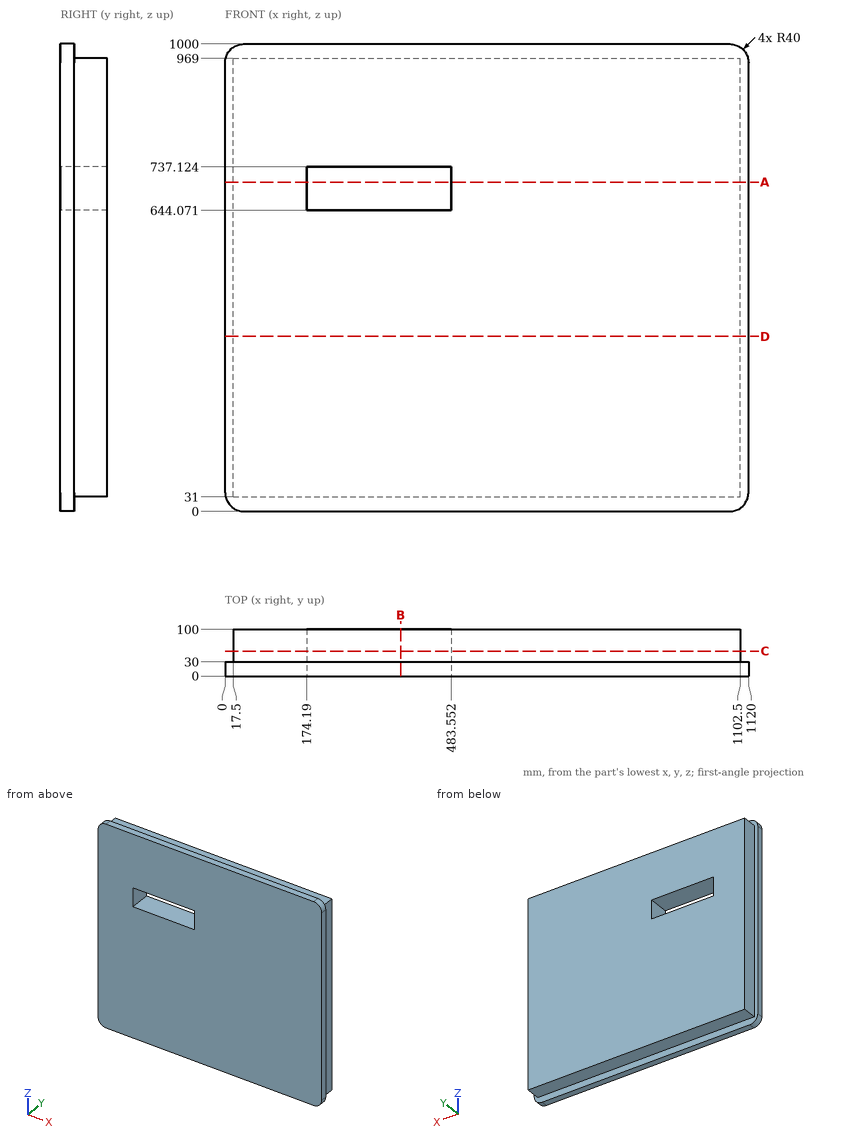
Study the drawing (mm; zero at the part's minimum x, y, z) and answer. Coordinates: 2 decimals unless noted, no trailing zeros. Write each loop counter-clockwise with the first axis right and the second up, starting at its lowest first coordinate (ties: lowest second). Pieces come first, ordered by that corner, then holes. Notation, with made-up numbers: (-39, 81.25) - (-21, 81.25) arc R17 ccw to (-21, 99.25) - close; hole circle Ø8 at (88, 24.5). An arc over 180 degrees is marked (long way). Answer as a JSON object with one key per item and string values.
Q1. Consider L1, parallel to Z at x = 228.5, y = 86; L2, parallel to X at y = 73, z = 665; L3, parallel to X at y = 60.5, z = 99. Determine where each line is inside the solid, lowest interval first. Write a range as from..to.
Results list:
{"L1": "z = 31..644.07, 737.12..969", "L2": "x = 17.5..174.19, 483.55..1102.5", "L3": "x = 17.5..1102.5"}
Q2. Find section D-D (z = 374.5). Write down the section's boundary in (x, y), plus the area to 3 significant figures.
Results list:
{"outline": "(0, 0) - (1120, 0) - (1120, 30) - (1102.5, 30) - (1102.5, 100) - (17.5, 100) - (17.5, 30) - (0, 30) - close", "area": "110,000 mm^2"}
Q3. Find section A-A (z = 704.5). Write down the section's boundary in (x, y), plus the area to 3 significant figures.
Results list:
{"outline": "(0, 0) - (174.19, 0) - (174.19, 100) - (17.5, 100) - (17.5, 30) - (0, 30) - close; (483.55, 0) - (1120, 0) - (1120, 30) - (1102.5, 30) - (1102.5, 100) - (483.55, 100) - close", "area": "78,600 mm^2"}
Q4. Given pin 1 Ø4 at (y, z) = (38.5, 745.5) entering from -X; pin 2 Ø4 at (x, y) = (715.5, 59.5) entering from -Z; pin 3 Ø6 at (y, z) = (63.5, 174.5) entering from +X, each flat-ended and moving along its own axis, determine where each tip first touches the part or whether it passes through.
Results list:
{"pin 1": "stops at x = 17.5", "pin 2": "stops at z = 31", "pin 3": "stops at x = 1102.5"}
Q5. Find section C-C (y = 53.5). Write down the section's boundary in (x, z), plus the area to 3 significant figures.
Results list:
{"outline": "(17.5, 31) - (1102.5, 31) - (1102.5, 969) - (17.5, 969) - close; hole (174.19, 644.07) - (483.55, 644.07) - (483.55, 737.12) - (174.19, 737.12) - close", "area": "989,000 mm^2"}
Q6. Find section B-B (x = 375.5). Write down the section's boundary in (y, z).
Results list:
{"outline": "(0, 0) - (30, 0) - (30, 31) - (100, 31) - (100, 644.07) - (0, 644.07) - close; (0, 737.12) - (100, 737.12) - (100, 969) - (30, 969) - (30, 1000) - (0, 1000) - close"}
